Input: part model. Units: mm. Frame: model coordinates. A direction names the side the tool comes from. Give positions to 0.01 mm unless a question says otherwise; leave off trailing zeros.
```python
from build123d import *

# Parameters (mm, degrees)
SKETCH1_W                = 50
SKETCH1_H                = 21
BOSS_EXTRUDE1_DEPTH      = 58
SKETCH3_R                = 7.5
CUT_EXTRUDE1_DEPTH       = 24
CUT_EXTRUDE2_REACH       = 66.025
SKETCH4_R                = 5.2
CUT_EXTRUDE3_START       = -24
SKETCH5_R                = 7.5
CUT_EXTRUDE3_DEPTH       = 24
CUT_EXTRUDE4_REACH       = 66.025
SKETCH6_R                = 4.5
CUT_EXTRUDE5_REACH       = 68.558
SKETCH8_W                = 10
SKETCH8_H                = 18
SKETCH9_W                = 5
SKETCH9_H                = 58
BOSS_EXTRUDE3_DEPTH      = 48
CUT_EXTRUDE7_REACH       = 95.916
BOSS_EXTRUDE4_START      = -25
BOSS_EXTRUDE4_OUTLINE_W  = 4
BOSS_EXTRUDE4_OUTLINE_H  = 48
BOSS_EXTRUDE4_DEPTH      = 50.0000001
BOSS_EXTRUDE4_2_DEPTH    = 4
SKETCH7_R                = 4.1
CUT_EXTRUDE8_DEPTH       = 15
SKETCH19_R               = 1.95
CUT_EXTRUDE11_DEPTH      = 10
CUT_EXTRUDE12_DEPTH      = 87.088617327
CUT_EXTRUDE12_DEPTH_BACK = 87.088617327
SKETCH20_W               = 5.527864045
SKETCH20_H               = 1
BOSS_EXTRUDE5_DEPTH      = 13
CUT_EXTRUDE13_START      = -69
CUT_EXTRUDE13_DEPTH      = 69
CUT_EXTRUDE14_REACH      = 90.833
SKETCH23_R               = 3.5
BOSS_EXTRUDE7_DEPTH      = 11
CUT_EXTRUDE15_REACH      = 98.074
SKETCH26_R               = 3.5
CUT_EXTRUDE16_DEPTH      = 15
FILLET1_R                = 5


with BuildPart() as part:
    # Sketch1 → Boss-Extrude1 (new body)
    with BuildSketch(Plane(origin=(0, 0, 0), x_dir=(1, 0, 0), z_dir=(0, 1, 0))):
        Rectangle(SKETCH1_W, SKETCH1_H)
    extrude(amount=BOSS_EXTRUDE1_DEPTH)

    # Sketch3 → Cut-Extrude1 (cut)
    with BuildSketch(Plane(origin=(0, 58, 0), x_dir=(1, 0, 0), z_dir=(0, 1, 0))):
        with Locations(Location((-15, 0, 0), (0, 0, 270))):
            Circle(SKETCH3_R)
    extrude(amount=-CUT_EXTRUDE1_DEPTH, mode=Mode.SUBTRACT)

    # Sketch4 → Cut-Extrude2 (cut, up to next)
    with BuildSketch(Plane(origin=(0, 58, 0), x_dir=(1, 0, 0), z_dir=(0, 1, 0)), mode=Mode.PRIVATE) as cut_extrude2_sk1:
        with Locations(Location((15, 0, 0), (0, 0, 270))):
            Circle(SKETCH4_R)
    cut_extrude2_tool1 = extrude(cut_extrude2_sk1.sketch, amount=-CUT_EXTRUDE2_REACH, mode=Mode.PRIVATE) & part.part
    add(cut_extrude2_tool1.solids().sort_by_distance((15, 58, 0))[0], mode=Mode.SUBTRACT)

    # Sketch5 → Cut-Extrude3 (cut)
    with BuildSketch(Plane.XZ.offset(CUT_EXTRUDE3_START)):
        with Locations(Location((-15, 0, 0), (0, 0, 90))):
            Circle(SKETCH5_R)
    extrude(amount=CUT_EXTRUDE3_DEPTH, mode=Mode.SUBTRACT)

    # Sketch6 → Cut-Extrude4 (cut, up to next)
    with BuildSketch(Plane.XZ, mode=Mode.PRIVATE) as cut_extrude4_sk1:
        with Locations(Location((-15, 0, 0), (0, 0, 270))):
            Circle(SKETCH6_R)
    cut_extrude4_tool1 = extrude(cut_extrude4_sk1.sketch, amount=-CUT_EXTRUDE4_REACH, mode=Mode.PRIVATE) & part.part
    add(cut_extrude4_tool1.solids().sort_by_distance((-15, 0, 0))[0], mode=Mode.SUBTRACT)

    # Sketch8 → Cut-Extrude5 (cut, up to next)
    with BuildSketch(Plane.XY.offset(10.5), mode=Mode.PRIVATE) as cut_extrude5_sk1:
        with Locations((0, 29)):
            Rectangle(SKETCH8_W, SKETCH8_H)
    cut_extrude5_tool1 = extrude(cut_extrude5_sk1.sketch, amount=-CUT_EXTRUDE5_REACH, mode=Mode.PRIVATE) & part.part
    add(cut_extrude5_tool1.solids().sort_by_distance((0, 29, 10.5))[0], mode=Mode.SUBTRACT)

    # Sketch9 → Boss-Extrude3 (add)
    with BuildSketch(Plane(origin=(0, 0, -10.5), x_dir=(-1, 0, 0), z_dir=(0, 0, -1))):
        with Locations((17.6, 29)):
            Rectangle(SKETCH9_W, SKETCH9_H)
    extrude(amount=BOSS_EXTRUDE3_DEPTH)

    # Sketch10 → Cut-Extrude7 (cut, up to next)
    with BuildSketch(Plane.ZY.offset(20.1), mode=Mode.PRIVATE) as cut_extrude7_sk1:
        with BuildLine():
            Line((-46.5, 46.2), (-53.5, 46.2))
            ThreePointArc((-53.5, 46.2), (-55.25, 44.45), (-53.5, 42.7))
            Line((-53.5, 42.7), (-46.5, 42.7))
            ThreePointArc((-46.5, 42.7), (-44.75, 44.45), (-46.5, 46.2))
        make_face()
    cut_extrude7_tool1 = extrude(cut_extrude7_sk1.sketch, amount=-CUT_EXTRUDE7_REACH, mode=Mode.PRIVATE) & part.part
    # Sketch10 → Cut-Extrude7 (cut, up to next)
    with BuildSketch(Plane.ZY.offset(20.1), mode=Mode.PRIVATE) as cut_extrude7_sk2:
        with BuildLine():
            Line((-41.5, 17), (-27.5, 17))
            ThreePointArc((-27.5, 17), (-23.964466094, 18.464466094), (-22.5, 22))
            Line((-22.5, 22), (-22.5, 36))
            ThreePointArc((-22.5, 36), (-23.964466094, 39.535533906), (-27.5, 41))
            Line((-27.5, 41), (-41.5, 41))
            ThreePointArc((-41.5, 41), (-45.035533906, 39.535533906), (-46.5, 36))
            Line((-46.5, 36), (-46.5, 22))
            ThreePointArc((-46.5, 22), (-45.035533906, 18.464466094), (-41.5, 17))
        make_face()
    cut_extrude7_tool2 = extrude(cut_extrude7_sk2.sketch, amount=-CUT_EXTRUDE7_REACH, mode=Mode.PRIVATE) & part.part
    # Sketch10 → Cut-Extrude7 (cut, up to next)
    with BuildSketch(Plane.ZY.offset(20.1), mode=Mode.PRIVATE) as cut_extrude7_sk3:
        with BuildLine():
            Line((-15.5, 15.3), (-22.5, 15.3))
            ThreePointArc((-22.5, 15.3), (-24.25, 13.55), (-22.5, 11.8))
            Line((-22.5, 11.8), (-15.5, 11.8))
            ThreePointArc((-15.5, 11.8), (-13.75, 13.55), (-15.5, 15.3))
        make_face()
    cut_extrude7_tool3 = extrude(cut_extrude7_sk3.sketch, amount=-CUT_EXTRUDE7_REACH, mode=Mode.PRIVATE) & part.part
    # Sketch10 → Cut-Extrude7 (cut, up to next)
    with BuildSketch(Plane.ZY.offset(20.1), mode=Mode.PRIVATE) as cut_extrude7_sk4:
        with BuildLine():
            Line((-46.5, 11.8), (-53.5, 11.8))
            ThreePointArc((-53.5, 11.8), (-55.25, 13.55), (-53.5, 15.3))
            Line((-53.5, 15.3), (-46.5, 15.3))
            ThreePointArc((-46.5, 15.3), (-44.75, 13.55), (-46.5, 11.8))
        make_face()
    cut_extrude7_tool4 = extrude(cut_extrude7_sk4.sketch, amount=-CUT_EXTRUDE7_REACH, mode=Mode.PRIVATE) & part.part
    # Sketch10 → Cut-Extrude7 (cut, up to next)
    with BuildSketch(Plane.ZY.offset(20.1), mode=Mode.PRIVATE) as cut_extrude7_sk5:
        with BuildLine():
            Line((-15.5, 46.2), (-22.5, 46.2))
            ThreePointArc((-22.5, 46.2), (-24.25, 44.45), (-22.5, 42.7))
            Line((-22.5, 42.7), (-15.5, 42.7))
            ThreePointArc((-15.5, 42.7), (-13.75, 44.45), (-15.5, 46.2))
        make_face()
    cut_extrude7_tool5 = extrude(cut_extrude7_sk5.sketch, amount=-CUT_EXTRUDE7_REACH, mode=Mode.PRIVATE) & part.part
    add(cut_extrude7_tool1.solids().sort_by_distance((-20.1, 44.45, -50))[0], mode=Mode.SUBTRACT)
    add(cut_extrude7_tool2.solids().sort_by_distance((-20.1, 29, -34.5))[0], mode=Mode.SUBTRACT)
    add(cut_extrude7_tool3.solids().sort_by_distance((-20.1, 13.55, -19))[0], mode=Mode.SUBTRACT)
    add(cut_extrude7_tool4.solids().sort_by_distance((-20.1, 13.55, -50))[0], mode=Mode.SUBTRACT)
    add(cut_extrude7_tool5.solids().sort_by_distance((-20.1, 44.45, -19))[0], mode=Mode.SUBTRACT)

    # Boss-Extrude4: read off the stored shape, not the designer's step
    # Boss-Extrude4 outline → Boss-Extrude4 (add)
    with BuildSketch(Plane.YZ.offset(BOSS_EXTRUDE4_START)):
        with Locations((2, -34.5)):
            Rectangle(BOSS_EXTRUDE4_OUTLINE_W, BOSS_EXTRUDE4_OUTLINE_H)
    boss_extrude4 = extrude(amount=BOSS_EXTRUDE4_DEPTH)

    # Boss-Extrude4 2 outline → Boss-Extrude4 2 (cut)
    with BuildSketch(Plane(origin=(0, 0, 0), x_dir=(1, 0, 0), z_dir=(0, 1, 0))):
        with BuildLine():
            Line((25.0000001, 58.5), (-15.1, 58.5))
            add(Edge.make_bspline(
                [(-15.1, 58.5), (-15.109460691, 13.119942058), (0.853801952, 10.552902486), (25, 10.5)],
                knots=[0, 0, 0, 0, 1, 1, 1, 1], degree=3))
            Line((25, 10.5), (25.0000001, 58.5))
        make_face()
        with BuildLine():
            ThreePointArc((-25, 55.5), (-24.121320344, 57.621320344), (-22, 58.5))
            Line((-22, 58.5), (-25, 58.5))
            Line((-25, 58.5), (-25, 55.5))
        make_face()
    boss_extrude4_2 = extrude(amount=BOSS_EXTRUDE4_2_DEPTH, mode=Mode.SUBTRACT)

    # Mirror1: Boss-Extrude4, Boss-Extrude4 2 across plane
    add(boss_extrude4.mirror(Plane(origin=(0, 29, 0), x_dir=(0, 0, 1), z_dir=(0, -1, 0))))
    add(boss_extrude4_2.mirror(Plane(origin=(0, 29, 0), x_dir=(0, 0, 1), z_dir=(0, -1, 0))), mode=Mode.SUBTRACT)

    # Sketch7 → Cut-Extrude8 (cut)
    with BuildSketch(Plane.XY.offset(10.5)):
        with Locations((0, 49)):
            Circle(SKETCH7_R)
        with Locations(Location((0, 9, 0), (0, 0, 180))):
            Circle(SKETCH7_R)
    extrude(amount=-CUT_EXTRUDE8_DEPTH, mode=Mode.SUBTRACT)

    # Sketch19 → Cut-Extrude11 (cut)
    with BuildSketch(Plane(origin=(0, 58, 0), x_dir=(1, 0, 0), z_dir=(0, 1, 0))):
        with Locations(Location((20.550788232, 5.550788232, 0), (0, 0, 270))):
            Circle(SKETCH19_R)
        with Locations(Location((9.449211768, -5.550788232, 0), (0, 0, 270))):
            Circle(SKETCH19_R)
    extrude(amount=-CUT_EXTRUDE11_DEPTH, mode=Mode.SUBTRACT)

    # Sketch20 → Cut-Extrude12 (cut, two sides: drawn at the far end of the back side and taken through both)
    with BuildSketch(Plane.XZ.offset(-CUT_EXTRUDE12_DEPTH_BACK)):
        with Locations((-22.236067977, 0)):
            Rectangle(SKETCH20_W, SKETCH20_H)
    extrude(amount=CUT_EXTRUDE12_DEPTH + CUT_EXTRUDE12_DEPTH_BACK, mode=Mode.SUBTRACT)

    # Sketch21 → Boss-Extrude5 (add)
    with BuildSketch(Plane(origin=(25, 0, 0), x_dir=(0, 0, -1), z_dir=(1, 0, 0))):
        Polygon((10.5, 0), (10.5, 58), (-10.5, 58), (-10.5, 0), (-7.5, 0), (-7.5, 55), (7.5, 55), (7.5, 0), align=None)
    extrude(amount=BOSS_EXTRUDE5_DEPTH)

    # Sketch22 → Cut-Extrude13 (cut)
    with BuildSketch(Plane.XY.offset(10.5).offset(CUT_EXTRUDE13_START)):
        with BuildLine():
            Line((25, 0), (38, 0))
            Line((38, 0), (38, 55))
            add(Edge.make_bspline(
                [(38, 55), (31.45567161, 55), (25, 40.968536323), (25, 0)],
                knots=[0, 0, 0, 0, 1, 1, 1, 1], degree=3))
        make_face()
    extrude(amount=CUT_EXTRUDE13_DEPTH, mode=Mode.SUBTRACT)

    # Sketch23 → Cut-Extrude14 (cut, up to next)
    with BuildSketch(Plane.XZ.offset(-55), mode=Mode.PRIVATE) as cut_extrude14_sk1:
        with Locations(Location((32.5, 0, 0), (0, 0, 270))):
            Circle(SKETCH23_R)
    cut_extrude14_tool1 = extrude(cut_extrude14_sk1.sketch, amount=-CUT_EXTRUDE14_REACH, mode=Mode.PRIVATE) & part.part
    add(cut_extrude14_tool1.solids().sort_by_distance((32.5, 55, 0))[0], mode=Mode.SUBTRACT)

    # Sketch24 → Boss-Extrude7 (add)
    with BuildSketch(Plane.XZ):
        Polygon((7.5, 10.5), (7.5, -11.859875449), (5, -11.859875449), (5, 8), (-5, 8), (-5, -11.859875449), (-7.5, -11.859875449), (-7.5, 10.5), align=None)
    extrude(amount=BOSS_EXTRUDE7_DEPTH)

    # Sketch26 → Cut-Extrude15 (cut, up to next)
    with BuildSketch(Plane(origin=(0, 0, 8), x_dir=(-1, 0, 0), z_dir=(0, 0, -1)), mode=Mode.PRIVATE) as cut_extrude15_sk1:
        with Locations((0, -5.5)):
            Circle(SKETCH26_R)
    cut_extrude15_tool1 = extrude(cut_extrude15_sk1.sketch, amount=-CUT_EXTRUDE15_REACH, mode=Mode.PRIVATE) & part.part
    add(cut_extrude15_tool1.solids().sort_by_distance((0, -5.5, 8))[0], mode=Mode.SUBTRACT)

    # Sketch27 → Cut-Extrude16 (cut)
    with BuildSketch(Plane.ZY.offset(7.5)):
        with BuildLine():
            Line((8, -11), (-11.859875449, -11))
            Line((-11.859875449, -11), (-11.859875449, 0))
            add(Edge.make_bspline(
                [(8, -11), (8, -5.603660731), (0.903317246, 0), (-11.859875449, 0)],
                knots=[0, 0, 0, 0, 1, 1, 1, 1], degree=3))
        make_face()
    extrude(amount=-CUT_EXTRUDE16_DEPTH, mode=Mode.SUBTRACT)

    # Fillet1
    # the kernel refuses this fillet: 5 mm, written as the material it takes off along each edge
    with BuildSketch(Plane(origin=(-25, -12.5, 10.5), x_dir=(1, 0, 0), z_dir=(0, 1, 0))) as fillet1_piece_1:
        with BuildLine():
            CenterArc((FILLET1_R, FILLET1_R), FILLET1_R, 180, 90)
            Line((0, FILLET1_R), (0, 0))
            Line((0, 0), (FILLET1_R, 0))
        make_face()
    extrude(amount=83, mode=Mode.SUBTRACT)
    with BuildSketch(Plane(origin=(38, 70.5, 10.5), x_dir=(-1, 0, 0), z_dir=(0, -1, 0)), Plane(origin=(38, 42.5, -10.5), x_dir=(-1, 0, 0), z_dir=(0, 1, 0))) as fillet1_piece_2:
        with BuildLine():
            CenterArc((FILLET1_R, FILLET1_R), FILLET1_R, 180, 90)
            Line((0, FILLET1_R), (0, 0))
            Line((0, 0), (FILLET1_R, 0))
        make_face()
    extrude(amount=28, mode=Mode.SUBTRACT)
    with BuildSketch(Plane(origin=(-7.5, -11, -4.5), x_dir=(1, 0, 0), z_dir=(0, 0, 1))) as fillet1_piece_3:
        with BuildLine():
            CenterArc((FILLET1_R, FILLET1_R), FILLET1_R, 180, 90)
            Line((0, FILLET1_R), (0, 0))
            Line((0, 0), (FILLET1_R, 0))
        make_face()
    extrude(amount=27.5, mode=Mode.SUBTRACT)
    with BuildSketch(Plane(origin=(7.5, -11, 23), x_dir=(0, 1, 0), z_dir=(0, 0, -1))) as fillet1_piece_4:
        with BuildLine():
            CenterArc((FILLET1_R, -FILLET1_R), FILLET1_R, 90, 90)
            Line((0, -FILLET1_R), (0, 0))
            Line((0, 0), (FILLET1_R, 0))
        make_face()
    extrude(amount=27.5, mode=Mode.SUBTRACT)


solid = part.part
```
Q1. Access query for faces 5 (the flat face through (28, 44, -7.5)), 6 (the flat face through (20, 0, -3)), 7 (the flat face through (0, 20, 0)), 8 (the flat face through (-18, 11.8, -19)), 9 (the flat face through (0.1, -1.8, 8)). Directions: +Z, -Z, +X, -X, +Y, -Y. A direction counts if a zero-diameter tool reaches every point of the face in a straight line with its end or side. Return the directions, or none.
Q2. Mould query, pull axis Z, two halves, no side actions, for faces 1 (the flat face through (-18, 15.3, -50)), 2 (the cylindrical face through (35.913, 56.346, 9.564)), 3 (the flat face through (5, -2, 3)), 4 (the flat face through (9, 48, 6)). Classes: +Z half, -Z half, draft (parallel to the pull), parting line (faces both ways), or undercut.
Q3. Material intervals for line 1 along Y through (x, z) = (0, 9.45); line 2 along X through (y, z) = (9, 0); line 3 along Y through (x, z) = (0, 5), sorted ascending.
Q4. Section A-A, the plane y = 30. Give the number of separate pieces and of enclosed holes in the cut face, then the cut area to 3 significant figures.
Q5. Pin query (flat end, axial travel): pin 1 (2 mm diameter, centred on y = 14.5, z = -41, fed in from -X); pin 2 (6.5 mm diameter, centred on y = -2, z = -4, fed in from -X); pin 3 (19.5 mm diameter, centred on x = 12.5, z = -1, fed in from -Y); pin 4 (17 mm diameter, centred on x = -15, z = 0, fed in from -Y). Return the tip coordinate at first contact, or that it passes through.
Solutions:
1. face 5: +X, -Y
1. face 6: +Z, -Z, +X, -Y
1. face 7: +Z, -Z
1. face 8: +X, -X
1. face 9: -Z, -Y
2. face 1: undercut
2. face 2: +Z half
2. face 3: draft
2. face 4: undercut
3. line 1: y = -11 to -9, -2 to 4.9, 13.1 to 20, 38 to 44.9, 53.1 to 58
3. line 2: x = -7.5 to -4.1, 4.1 to 9.8, 20.2 to 25
3. line 3: y = 0 to 4.9, 13.1 to 20, 38 to 44.9, 53.1 to 58
4. separate pieces: 3
4. enclosed holes: 1
4. area: 810 mm2
5. pin 1: stops at x = -20.1
5. pin 2: stops at x = -25
5. pin 3: stops at y = -7.79
5. pin 4: stops at y = -4.25
